For this review, take the finished solid that the model builds, in its own axes (mm). A direction names the side the tool comes from. Give positions to 0.01 mm unless a question says otherwise; leave off trailing zeros. Loops run counter-clockwise (first coordinate to the right, second up) from the corner with the lowest first, then second, coordinate; pieces in that order, holes last. Notation, with made-up numbers: (-26, 41.5) -> (6, 41.5) arc R15 ccw to (6, 68.5) -> close; hole circle Ø11 at (-10, 76). An arc over 180 degrees is marked (long way). Answer as CSV lines item,"result". Start each with the question number.
Item 1: Add section C-C on z = -77. State the section outline as (x, y) points.
Item 2: Machinability: for faces 1 (the face through (61.5, 73.253, 3.183)), 2 (the face through (66, 75, -107.95)), which of the approach directions +Z, -Z, +X, -X, +Y, -Y give a long, thin tool a straight path to every point of the face, cutting with its end or side? Answer none if there is none.
Item 3: Clearance check with flat-ended pins moving along their axes: P1, Ø1, axis at x = 48, z = -42.5, coming from the +Y side; P2, Ø2, axis at x = 17.5, z = -7.5, coming from the -Y side; P3, Ø5, axis at x = 67, z = -19, coming from the +Y side. State where each tip first meets the part, or that it passes through.
Item 4: Add section B-B on z = -16. State the section outline as (x, y) points, plus the area to 3 significant figures.
Item 5: For L1, parallel to Z at x = -16, y = 34; L2, parallel to X at y = 103.5, z = -44; L3, parallel to X at y = 102, z = -71.5, list the stretches that pass through material, from the lowest coordinate up. Write a range as from..to.
Item 6: Add section A-A on y = 48.5. State how many separate pieces and enclosed holes the cut face has, plus the area to 3 significant figures.
Item 7: The part is to be moulded in two halves that separate along Z. For faces 3 (the face through (-45, 0, -54)), 4 (the face through (66, 75, 0)), 5 (the face through (66, 75, -114.407)), say which applies: +Z half, -Z half, draft (parallel to the pull), parting line (faces both ways), or undercut.
Autodesk Inventor part; units mm, degrees
ref_plane "YZ Plane" through (0, 0, 0) normal (1, 0, 0) x (0, 1, 0)
ref_plane "XZ Plane" through (0, 0, 0) normal (0, 1, 0) x (-1, 0, 0)
ref_plane "XY Plane" through (0, 0, 0) normal (0, 0, 1) x (1, 0, 0)
sketch "Sketch2" plane through (0, 0, 0) normal (0, 1, 0) x (-1, 0, 0)
  line L0 (0, 0) -> (0, -107.95) construction
  line L1 (0, -53.975) -> (44.45, -53.975) construction
  arc A0 (0, -107.95) -> (0, 0) centre (-10.5455, -53.975) ccw
  arc A1 (0, -114.4073) -> (0, 6.4573) centre (-10.5455, -53.975) ccw
  line L2 (0, 0) -> (0, 6.4573)
  line L3 (0, -107.95) -> (0, -114.4073)
  line L4 (0, 6.4573) -> (-6.35, 6.4573)
  line L5 (-6.35, 6.4573) -> (-6.35, 0)
  line L6 (-6.35, 0) -> (0, 0)
  line L7 (0, 0) -> (0, 6.4573)
  line L8 (0, -107.95) -> (-6.35, -107.95)
  line L9 (-6.35, -107.95) -> (-6.35, -114.4073)
  line L10 (-6.35, -114.4073) -> (0, -114.4073)
  line L11 (0, -114.4073) -> (0, -107.95)
  line L12 (44.45, -53.975) -> (-82.55, -53.975) construction
  line L13 (-82.5742, -64.2808) -> (-82.5742, -44.6455) construction
  dimension "d5" = 107.95
  dimension "d6" = 44.45
  dimension "d7" = 6.35
  dimension "d8" = 6.35
  dimension "d9" = 127
revolve "Revolution2" add sketch "Sketch2" angle 150 about axis through (82.5742, 0, -64.2808) along (0, 0, -1)
properties part number "throwerRamp"
Computed values:
1,outline,"(-46.32, 0) -> (-39.4, 0) arc R121.97 cw to (188.21, 60.99) -> (194.2, 64.44) arc R128.89 ccw to start"
2,face 1,"+Z, -Z, -Y"
2,face 2,"-Y"
3,P1,"y = 127.86"
3,P2,"y = 75.49"
3,P3,"y = 123.12"
4,outline,"(-37.63, 0) -> (-29.23, 0) arc R111.81 cw to (179.4, 55.9) -> (186.68, 60.1) arc R120.21 ccw to start"
4,area,"2,550 mm²"
5,L1,"-106.16..-98.53, -9.42..-1.79"
5,L2,"-0.25..10.52, 154.63..165.4"
5,L3,"0.66..11.79, 153.36..164.48"
6,separate pieces,"3"
6,enclosed holes,"0"
6,area,"1,580 mm²"
7,face 3,"draft"
7,face 4,"undercut"
7,face 5,"-Z half"
